For this review, use the dimensioned drawing (mm, ordinates from the lowest corner) and the shaded views. A direction names the side the tool comes from. Round coordinates to 2 decimals unless told otherwise and drop trailing zeros. Loops run counter-clockwise (first coordinate to the right, second up) from the corner with the lowest first, then second, coordinate; pieces in that order, holes last. Notation, with made-up numbers: M 15.25,88.25 L 61.25,88.25 A15 cw 61.25,114.25 Z; hole C 27.5,39.25 d9. An arc over 180 degrees is marked long. Answer as a JSON object with one key per item and string values. Group by question number.
Item 1: Tool access review of the marked faces 5 and 6: name each direction out of +Z, -Z, +X, -X, +Y, -Y from which nothing blocks a thin tool from reaching the whole face with its end or side.
Item 2: Consider section A-A (z = 6). Give the boundary of the cut face in (x, y) (3 decimals).
Item 3: Consider section C-C (x = 5.25). Give the boundary of the cut face in (y, z), and give its area (4 significant figures).
Item 4: Insertion check: P1, Ø1.5, axis at x = 11.5, z = 1.5, coming from the -Y side. The pin has a flat end and moves straight along its axis. Give the tip position at first contact, or say it passes through.
Item 5: The part is to be moulded in two halves that separate along X. For the marked faces 1, 2, 3 and 4, say which applies: +X half, -X half, draft (parallel to the pull), parting line (faces both ways), or undercut.
Item 6: Consider section B-B (y = 1.8). Give the boundary of the cut face in (x, z) (3 decimals), and give its area (3 significant figures).
Item 7: Consider section D-D (y = 3.7). Give the boundary of the cut face in (x, z) (3 decimals), and give its area (3 significant figures).
Item 8: To check wall thickness, follow line 1 (X direction, y = 1.25, z = 9); line 2 (X direction, y = 1.5, z = 8); line 3 (Y direction, x = 3.5, z = 10.75). State the ranges of each line that lie inside material, in increasing order.
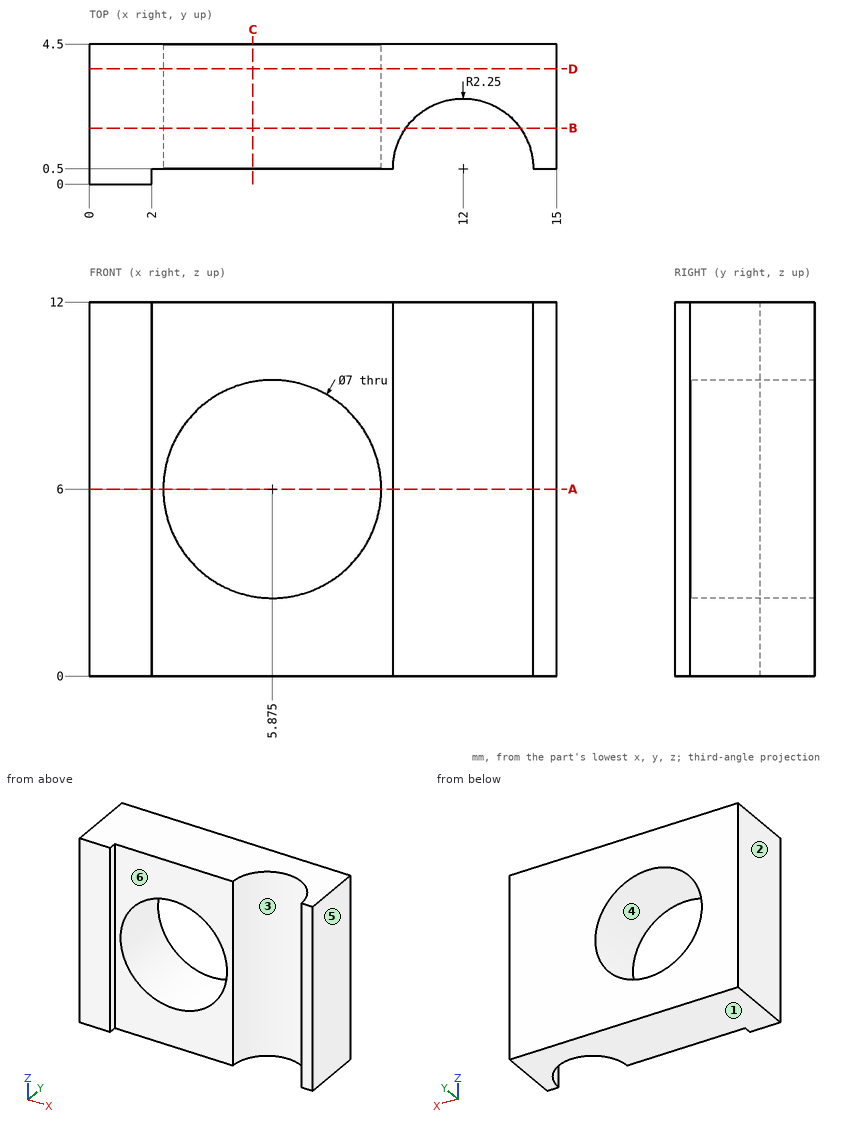
Geometry results:
{
 "1": {"face 5": "+Z, -Z, +X, +Y, -Y", "face 6": "+Z, -Z, +X, -Y"},
 "2": {"outline": "M 0,0 L 2,0 L 2,0.5 L 2.375,0.5 L 2.375,4.5 L 0,4.5 Z; M 9.375,0.5 L 9.75,0.5 A2.25 cw 14.25,0.5 L 15,0.5 L 15,4.5 L 9.375,4.5 Z"},
 "3": {"outline": "M 0.5,0 L 4.5,0 L 4.5,2.56 L 0.5,2.56 Z; M 0.5,9.44 L 4.5,9.44 L 4.5,12 L 0.5,12 Z", "area": "20.45 mm^2"},
 "4": {"P1": "stops at y = 2.37"},
 "5": {"face 1": "draft", "face 2": "-X half", "face 3": "undercut", "face 4": "undercut"},
 "6": {"outline": "M 0,0 L 10.164,0 L 10.164,12 L 0,12 Z; M 13.836,0 L 15,0 L 15,12 L 13.836,12 Z; hole C 5.875,6 d7", "area": "97.4 mm^2"},
 "7": {"outline": "M 0,0 L 15,0 L 15,12 L 0,12 Z; hole C 5.875,6 d7", "area": "142 mm^2"},
 "8": {"line 1": "x = 0 to 4.07, 7.68 to 9.88, 14.12 to 15", "line 2": "x = 0 to 3, 8.75 to 9.98, 14.02 to 15", "line 3": "y = 0.5 to 4.5"}
}
